```python
from build123d import *

# Parameters (mm, degrees)
F1_DEPTH  = 76.2
F2_R      = 20.701916
F3_DEPTH  = 63.501
F5_DEPTH  = 50.8
F7_DEPTH  = 114.301
F9_DEPTH  = 50.8
F11_DEPTH = 114.301
F12_W     = 22.93722
F12_H     = 45.488945
F13_DEPTH = 76.201


with BuildPart() as f1:
    # F0 (on Front) → F1 (new body)
    with BuildSketch(Plane.XZ):
        Polygon((-40.358745, -29.197829), (-40.358745, -54.597829), (48.541255, -54.597829), (48.541255, -29.197829), (23.141255, -29.197829), (23.141255, 34.302171), (48.541255, 34.302171), (48.541255, 59.702171), (-40.358745, 59.702171), (-40.358745, 34.302171), (-14.958745, 34.302171), (-14.958745, -29.197829), align=None)
    extrude(amount=F1_DEPTH)

    # F2 (on face) → F3 (cut, through all)
    with BuildSketch(Plane.YZ.offset(23.141255)):
        with Locations((-38.1, 2.552171)):
            Circle(F2_R)
    extrude(amount=-F3_DEPTH, mode=Mode.SUBTRACT)

    # F4 (on face) → F5 (join)
    with BuildSketch(Plane.XY.offset(59.702171)):
        Polygon((38.645647, -58.671612), (30.735792, -71.129635), (45.613699, -71.129635), align=None)
    extrude(amount=F5_DEPTH)

    # F6 (on face) → F7 (cut, through all)
    with BuildSketch(Plane.XY.offset(59.702171)):
        Polygon((-29.12768, -57.497039), (-34.554791, -69.002517), (-23.700567, -68.568349), align=None)
    extrude(amount=-F7_DEPTH, mode=Mode.SUBTRACT)

    # F8 (on face) → F9 (join)
    with BuildSketch(Plane.XY.offset(59.702171)):
        Polygon((-30.212333, -3.429755), (-35.322022, -13.198283), (-25.102641, -12.146287), align=None)
    extrude(amount=F9_DEPTH)

    # F10 (on face) → F11 (cut, through all)
    with BuildSketch(Plane.XY.offset(59.702171)):
        Polygon((41.774195, -5.233176), (38.167354, -14.701133), (46.433032, -14.701133), align=None)
    extrude(amount=-F11_DEPTH, mode=Mode.SUBTRACT)

    # F12 (on face) → F13 (cut, through all)
    with BuildSketch(Plane.XZ.offset(76.2)):
        with Locations((2.466541, 5.390951)):
            Rectangle(F12_W, F12_H)
    extrude(amount=-F13_DEPTH, mode=Mode.SUBTRACT)


solid = f1.part
```
Source: CAD feature listing. Evaluate the final solid. Frame: model axes, mm. A direction names the side the tool comes from. Round coordinates to 2 decimals unless told otherwise and drop trailing zeros. Write each loop counter-clockwise with the first axis right and the second up, starting at its lowest first coordinate (ties: lowest second). Pieces come first, ordered by that corner, then holes. Notation, with made-up numbers: M 24.5,25.5 L 34.5,25.5 A15 cw 34.5,33.5 Z; hole C 25,-34 d6. An arc over 180 degrees is marked long. Answer as a JSON object with one key per item and string values. Group by question number.
(1) Section query A-A on y = -38.1. Output: boundary loops of the cut face in (x, z), then the cut area to 3 significant figures.
(2) First-contact query: pin 1 (12 mm diameter, centred on x = 29.5, y = -53, fed in from +Z); pin 2 (12 mm diameter, centred on x = 40.5, z = 94.5, fed in from -Y); pin 3 (13.5 mm diameter, centred on y = -56, z = -1, fed in from +X). Flat tips, straight axial feed; report the tip coordinate or a pass-through.
(3) Section query D-D on z = 15.5. Output: boundary loops of the cut face in (x, y).
(4) Ray query, line 1 (Z direction, x = -16, y = -3.5); line 2 (Z direction, x = 9, y = -38.1); line 3 (X direction, y = -63.5, z = 9). Return the intervals inside material, ascending. Write a range as [from, to].
(5) Section query C-C on z = 71. Output: boundary loops of the cut face in (x, y), then the cut area to 3 significant figures.
(6) Mould query, pull axis X, two halves, no side actions, for faces 1 (the flat face through (39.996, -9.901, 47.18)), 2 (the flat face through (23.141, -38, -19)), 3 (the flat face through (3, -38, -54.598)), 4 (the flat face through (-14.959, -38, 24)). Classes: +X half, -X half, draft (parallel to the pull), parting line (faces both ways), or undercut.
(7) Section query B-B on x = -20. Output: boundary loops of the cut face in (y, z), then the cut area to 3 significant figures.
(8) Reachability of faces 5 (the flat face through (13.935, -56, 15)), 6 (the flat face through (36, -38, 34.302)), 7 (the flat face through (-27, -38, -29.198)), 8 (the flat face through (-30.28, -12.68, 84.75)), 9 (the flat face through (-31.803, -63.169, -41.72)) from +Z, -Z, +X, -X, +Y, -Y: full face, straight path, thin tool, end or side. Return the list, or none.
Computed values:
{
 "1": {"outline": "M -40.36,-54.6 L 48.54,-54.6 L 48.54,-29.2 L 23.14,-29.2 L 23.14,-18.15 L -14.96,-18.15 L -14.96,-29.2 L -40.36,-29.2 Z; M -40.36,34.3 L -14.96,34.3 L -14.96,23.25 L -9,23.25 L -9,28.14 L 13.94,28.14 L 13.94,23.25 L 23.14,23.25 L 23.14,34.3 L 48.54,34.3 L 48.54,59.7 L -40.36,59.7 Z", "area": "5,250 mm^2"},
 "2": {"pin 1": "z = 59.7", "pin 2": "y = -71.13", "pin 3": "x = 23.14"},
 "3": {"outline": "M -14.96,-76.2 L -9,-76.2 L -9,-54.25 L -14.96,-54.25 Z; M -14.96,-21.95 L -9,-21.95 L -9,0 L -14.96,0 Z; M 13.94,-76.2 L 23.14,-76.2 L 23.14,-54.25 L 13.94,-54.25 Z; M 13.94,-21.95 L 23.14,-21.95 L 23.14,0 L 13.94,0 Z"},
 "4": {"line 1": "[-54.6, -29.2], [34.3, 59.7]", "line 2": "[-54.6, -18.15], [28.14, 59.7]", "line 3": "[-14.96, -9], [13.94, 23.14]"},
 "5": {"outline": "M -35.32,-13.2 L -25.1,-12.15 L -30.21,-3.43 Z; M 30.74,-71.13 L 45.61,-71.13 L 38.65,-58.67 Z", "area": "140 mm^2"},
 "6": {"face 1": "undercut", "face 2": "+X half", "face 3": "draft", "face 4": "-X half"},
 "7": {"outline": "M -76.2,-54.6 L 0,-54.6 L 0,-29.2 L -76.2,-29.2 Z; M -76.2,34.3 L 0,34.3 L 0,59.7 L -76.2,59.7 Z", "area": "3,870 mm^2"},
 "8": {"face 5": "+Y, -Y", "face 6": "+X, +Y, -Y", "face 7": "-X, +Y, -Y", "face 8": "+Z, +X, -Y", "face 9": "+Z, -Z"}
}
